from build123d import *

# Parameters (mm, degrees)
BOSS_EXTRUDE2_DEPTH = 12.7
FILLET1_R           = 25.4
FILLET2_R           = 25.4
SKETCH3_R           = 3.175
CUT_EXTRUDE3_DEPTH  = 12.7


with BuildPart() as part:
    # Sketch1 → Boss-Extrude2 (new body)
    with BuildSketch(Plane.XY):
        with BuildLine():
            Line((0, 167.705976621), (0, 0))
            Line((0, 0), (-54.924735551, 0))
            Line((-54.924735551, 0), (-54.924735551, 254.93724428))
            Line((-54.924735551, 254.93724428), (105.37332707, 254.93724428))
            Line((105.37332707, 254.93724428), (105.37332707, 173.075661403))
            Line((105.37332707, 173.075661403), (105.37332707, 98.46451231))
            Line((105.37332707, 98.46451231), (50.448591519, 98.46451231))
            Line((50.448591519, 98.46451231), (50.448591519, 171.91644725))
            ThreePointArc((50.448591519, 171.91644725), (22.936036736, 197.228442673), (0, 167.705976621))
        make_face()
    extrude(amount=BOSS_EXTRUDE2_DEPTH)

    # Fillet1
    fillet1_edges = [part.edges().sort_by_distance(p)[0] for p in [
        (-54.924735551, 254.93724428, 6.35),
    ]]
    fillet(fillet1_edges, radius=FILLET1_R)

    # Fillet2
    fillet2_edges = [part.edges().sort_by_distance(p)[0] for p in [
        (105.37332707, 254.93724428, 6.35),
    ]]
    fillet(fillet2_edges, radius=FILLET2_R)

    # Sketch3 → Cut-Extrude3 (cut)
    with BuildSketch(Plane.XY.offset(12.7)):
        with Locations((-27.462367775, 30.26240116)):
            Circle(SKETCH3_R)
    extrude(amount=-CUT_EXTRUDE3_DEPTH, mode=Mode.SUBTRACT)


solid = part.part
Build history of the part. All positions in model axes, mm. A direction names the side the tool comes from. Give positions to 0.01 mm unless a question says otherwise; leave off trailing zeros. Loops run counter-clockwise (first coordinate to the right, second up) from the corner with the lowest first, then second, coordinate; pieces in that order, holes last. Notation, with made-up numbers: (39.5, -36) - (63.5, -36) arc R13 ccw to (63.5, -20) - close; hole circle Ø5 at (37.5, 46.25). An arc over 180 degrees is marked (long way). Write item = value, one per line. Start each with the question number.
1) Drop flat-ended pins along their axis: pin 1 Ø1.5 at (x, z) = (85.5, 10) entering from -Y; pin 2 Ø3 at (y, z) = (56, 3.5) entering from +X; pin 3 Ø5 at (x, z) = (11.5, 2) entering from -Y. Give the stop position or say it passes through.
2) Pull direction Y, two halves, no side cores. Call faces 4 (the flat face through (-27, 0, 6)), 5 (the flat face through (50.449, 135, 6)), 6 (the cylindrical face through (97.74, 247.69, 6.44)), 7 (the cylindrical face through (-27.88, 33.41, 6.44)): +Y half, -Y half, draft (parallel to the pull), parting line (faces both ways), or undercut.
3) Probe probe 1 along X at (y, z) = (138.5, 6.75); probe 2 along X at (y, z) = (47.5, 7.5); probe 3 along X at (y, z) = (171.5, 5.25). List the from-to ranges inside material, lowest first. Write a range as from..to.
4) Band-saw the part on B-B on z = 2.75. Give the cut face in (x, y) (3 decimals), plus the area to 3 significant figures.
5) Band-saw the part on C-C on y = 176. Give the cut face in (x, z), plus the area to 3 significant figures.
6) Tool access for faces 1 (the flat face through (105.373, 165, 6)), 2 (the flat face through (0, 85, 6)), 3 (the flat face through (78, 98.465, 6)): list every direction of +Z, -Z, +X, -X, +Y, -Y with a clear straight run to the whole face (end or side of a thin tool).
7) Band-saw the part on D-D on y = 89. Give the cut face in (x, z), plus the area to 3 significant figures.
8) Band-saw the part on A-A on y = 143. Give the cut face in (x, z), plus the area to 3 significant figures.
Final values:
q1.pin_1 = 98.46
q1.pin_2 = 0
q1.pin_3 = 191.6
q2.face_4 = -Y half
q2.face_5 = draft
q2.face_6 = +Y half
q2.face_7 = undercut
q3.probe_1 = -54.92..0, 50.45..105.37
q3.probe_2 = -54.92..0
q3.probe_3 = -54.92..-0.35, 50.45..105.37
q4.outline = (-54.925, 0) - (0, 0) - (0, 167.706) arc R25.4 cw (long way) to (50.449, 171.916) - (50.449, 98.465) - (105.373, 98.465) - (105.373, 229.537) arc R25.4 ccw to (79.973, 254.937) - (-29.525, 254.937) arc R25.4 ccw to (-54.925, 229.537) - close; hole circle Ø6.35 at (-27.462, 30.262)
q4.area = 25,500 mm²
q5.outline = (-54.92, 0) - (-0.02, 0) - (-0.02, 12.7) - (-54.92, 12.7) - close; (50.12, 0) - (105.37, 0) - (105.37, 12.7) - (50.12, 12.7) - close
q5.area = 1,400 mm²
q6.face_1 = +Z, -Z, +X, +Y, -Y
q6.face_2 = +Z, -Z, -Y
q6.face_3 = +Z, -Z, +X, -Y
q7.outline = (-54.92, 0) - (0, 0) - (0, 12.7) - (-54.92, 12.7) - close
q7.area = 698 mm²
q8.outline = (-54.92, 0) - (0, 0) - (0, 12.7) - (-54.92, 12.7) - close; (50.45, 0) - (105.37, 0) - (105.37, 12.7) - (50.45, 12.7) - close
q8.area = 1,400 mm²
